Input: part model. Units: mm. Frame: model coordinates. A direction names the side the tool comes from. Round coordinates to 2 decimals unless told otherwise and drop trailing zeros. Loops run counter-clockwise (first coordinate to the right, second up) from the corner with the lowest first, then second, coordinate; pieces in that order, holes last. Notation, with made-up numbers: M -20.75,-10.75 L 32.25,-10.75 A24 cw 32.25,5.25 Z; hole C 56,-19 d8. An arc over 180 degrees is marked long. Put each result on its own line as item: value. Start each with the question number.
1) Section A-A on z = -14.05. Output: boundary loops of the cut face in (x, y).
2) Reachability of faces 4 (the face through (8.02, 5.88, 3.39)), 5 (the face through (6, 0, -7)), 6 (the face through (6, -2, 11.55)), 7 (the face through (11, 0, 10)) from +Z, -Z, +X, -X, +Y, -Y: full face, straight path, thin tool, end or side. Return the list, or none.
3) Line query: probe 1 along X at (y, z) = (-4.85, 14.05); probe 2 along Y at (x, z) = (9.75, -6); probe 3 along Z at (x, y) = (7.5, -18.5). Output: solid intervals per line, ascending.
4) Draft query along X for faces 1 (the face through (6, -4.2, 13)), 2 (the face through (13, -11, 0)), 3 (the face through (6.47, -5.46, 13.05)). Return one class per face: +X half, -X half, draft (parallel to the pull), parting line (faces both ways), or undercut.
5) Section B-B on z = -1.45. Output: boundary loops of the cut face in (x, y).
6) Section D-D on y = -7.5. Output: boundary loops of the cut face in (x, z).
7) Section C-C on x = 9.5. Output: boundary loops of the cut face in (y, z).
8) Pin query (flat end, axial travel): pin 1 (3 mm diameter, centred on x = 10, z = 8, fed in from +Y); pin 2 (5 mm diameter, centred on x = 8.5, z = 1, fed in from +Y); pin 3 (1.3 mm diameter, centred on x = 6, y = -2, fed in from -Z); pin 4 (2.5 mm diameter, centred on x = 6.5, z = -14.05, fed in from +Y). Return the tip coordinate at first contact, or that it passes through.
from build123d import *

# Parameters (mm, degrees)
BOSS_EXTRUDE1_DEPTH = 13
BOSS_EXTRUDE2_DEPTH = 4.4
SKETCH3_R           = 2.25
BOSS_EXTRUDE3_DEPTH = 3
CUT_EXTRUDE1_REACH  = 30.22


with BuildPart() as part:
    # Sketch1 → Boss-Extrude1 (new body)
    with BuildSketch(Plane(origin=(0, 0, 0), x_dir=(0, 0, -1), z_dir=(1, 0, 0))):
        Polygon((11.55, -4.2), (16.55, -4.2), (16.55, -6.75), (11.55, -6.75), (11.55, -23), (-11.55, -23), (-11.55, -6.75), (-16.55, -6.75), (-16.55, -4.2), (-11.55, -4.2), (-11.55, 0), (11.55, 0), align=None)
    extrude(amount=BOSS_EXTRUDE1_DEPTH)

    # Sketch2 → Boss-Extrude2 (add)
    with BuildSketch(Plane(origin=(0, 0, 0), x_dir=(1, 0, 0), z_dir=(0, 1, 0))):
        with BuildLine():
            ThreePointArc((4.046663303, 0.969230769), (6.5, -11.55), (8.953336697, 0.969230769))
            ThreePointArc((8.953336697, 0.969230769), (6.5, 3.95), (4.046663303, 0.969230769))
        make_face()
    extrude(amount=BOSS_EXTRUDE2_DEPTH)

    # Sketch3 → Boss-Extrude3 (add)
    with BuildSketch(Plane(origin=(0, 4.4, 0), x_dir=(1, 0, 0), z_dir=(0, 1, 0))):
        with Locations(Location((6.5, -5.05, 0), (0, 0, 270))):
            Circle(SKETCH3_R)
    extrude(amount=BOSS_EXTRUDE3_DEPTH)

    # Sketch4 → Cut-Extrude1 (cut, up to next)
    with BuildSketch(Plane(origin=(0, -4.2, 0), x_dir=(1, 0, 0), z_dir=(0, 1, 0)), mode=Mode.PRIVATE) as cut_extrude1_sk1:
        with BuildLine():
            Line((5.75, -16.55), (5.75, -14.711437828))
            ThreePointArc((5.75, -14.711437828), (6.5, -13.05), (7.25, -14.711437828))
            Line((7.25, -14.711437828), (7.25, -16.55))
            Line((7.25, -16.55), (5.75, -16.55))
        make_face()
    cut_extrude1_tool1 = extrude(cut_extrude1_sk1.sketch, amount=-CUT_EXTRUDE1_REACH, mode=Mode.PRIVATE) & part.part
    cut_extrude1 = cut_extrude1_tool1.solids().sort_by_distance((6.5, -4.2, 14.785135))[0]
    add(cut_extrude1, mode=Mode.SUBTRACT)

    # Mirror1: Cut-Extrude1 across plane
    add(cut_extrude1.mirror(Plane.XY), mode=Mode.SUBTRACT)


solid = part.part
Geometry results:
1. outline: M 0,-6.75 L 5.5,-6.75 L 5.5,-4.2 L 0,-4.2 Z; M 7.5,-6.75 L 13,-6.75 L 13,-4.2 L 7.5,-4.2 Z
2. face 4: +Y
2. face 5: -Z, +Y
2. face 6: +Z, +X, -X, +Y
2. face 7: +Z, +X, +Y
3. probe 1: x = 0 to 5.5, 7.5 to 13
3. probe 2: y = -23 to 0
3. probe 3: z = -11.55 to 11.55
4. face 1: draft
4. face 2: +X half
4. face 3: undercut
5. outline: M 0,-23 L 13,-23 L 13,0 L 9,0 L 9,4.4 L 4,4.4 L 4,0 L 0,0 Z
6. outline: M 0,-11.55 L 13,-11.55 L 13,11.55 L 0,11.55 Z
7. outline: M -23,-11.55 L -6.75,-11.55 L -6.75,-16.55 L -4.2,-16.55 L -4.2,-11.55 L 0,-11.55 L 0,-0.72 L 4.4,-0.72 L 4.4,10.82 L 0,10.82 L 0,11.55 L -4.2,11.55 L -4.2,16.55 L -6.75,16.55 L -6.75,11.55 L -23,11.55 Z
8. pin 1: stops at y = 4.4
8. pin 2: stops at y = 7.4
8. pin 3: stops at z = -11.55
8. pin 4: stops at y = -4.2
